```python
from build123d import *

# Parameters (mm, degrees)
F0_R     = 30
F1_DEPTH = 0.5
F2_W     = 30
F2_H     = 1
F4_R     = 30
F4_R_2   = 29.5
F5_DEPTH = 23.5


with BuildPart() as f1:
    # F0 (on Top) → F1 (new body)
    with BuildSketch(Plane.XY):
        Circle(F0_R)
    extrude(amount=-F1_DEPTH)



with BuildPart() as f3:
    # F2 (on Front) → F3 (revolve)
    with BuildSketch(Plane.XZ):
        with Locations((15, -24.5)):
            Rectangle(F2_W, F2_H)
    revolve(axis=Axis((0, 0, -12.5), (0, 0, -1)))


with BuildPart() as f1_1:
    add(f1.part)

    add(f3.part)  # F5 merges F3
    # F4 (on face) → F5 (join, through all)
    with BuildSketch(Plane(origin=(0, 0, -0.5), x_dir=(1, 0, 0), z_dir=(0, 0, -1))):
        Circle(F4_R)
        Circle(F4_R_2, mode=Mode.SUBTRACT)
    extrude(amount=F5_DEPTH)


solid = f1_1.part
```
Build history of the part. All positions in model axes, mm. A direction names the side the tool comes from. Round coordinates to 2 decimals unless told otherwise and drop trailing zeros. Order: outer loops, then holes, each group sorted by start corner. A loop starts at its lowest first (then second) coordinate and runs counter-clockwise, first axis right, second up. Notation, with made-up numbers: (-7, 44) - (30, 44) arc R22 ccw to (30, 63) - close; hole circle Ø8 at (46.25, 45). An arc over 180 degrees is marked (long way). Use a Markdown table: item, result.
1) Saw through at A-A on y = 0. Write the cut outline in (x, z).
Recorded:
| item | result |
|---|---|
| outline | (-30, -25) - (30, -25) - (30, 0) - (-30, 0) - close; hole (-29.5, -24) - (29.5, -24) - (29.5, -0.5) - (-29.5, -0.5) - close |
2) Tool access for faces 1 (the face through (0, 0, -0.5)), 2 (the face through (0, 0, 0)): list every direction of +Z, -Z, +X, -X, +Y, -Y with a clear straight run to the whole face (end or side of a thin tool).
Recorded:
| item | result |
|---|---|
| face 1 | none |
| face 2 | +Z, +X, -X, +Y, -Y |
3) Flat gauge pins, fed straight in: pin 1 Ø6 at (x, z) = (-14.5, -12.5) entering from -Y; pin 2 Ø6 at (y, z) = (10, -19) entering from +X; pin 3 Ø6 at (y, z) = (8, -17.5) entering from -X; pin 4 Ø12 at (x, y) = (-10.5, 8) entering from +Z. Where does each tip first touch, or does it go through?
Recorded:
| item | result |
|---|---|
| pin 1 | stops at y = -27.71 |
| pin 2 | stops at x = 29.17 |
| pin 3 | stops at x = -29.58 |
| pin 4 | stops at z = 0 |
4) Saw through at C-C on z = -5. Write the cut outline in (x, y), and give its area (3 significant figures).
Recorded:
| item | result |
|---|---|
| outline | circle Ø60 at (0, 0); hole circle Ø59 at (0, 0) |
| area | 93.5 mm² |
5) Pull direction Y, two halves, no side cores. Call faces 3 (the face through (0, 0, -25)), 4 (the face through (0, 0, -24)), 5 (the face through (28.14, -8.86, -12.09)): pulls with the +Y half, pulls with the -Y half, needs draft (parallel to the pull), parting line crosses it, or undercut.
Recorded:
| item | result |
|---|---|
| face 3 | needs draft |
| face 4 | undercut |
| face 5 | undercut |
6) Wall check: L1, parallel to X at y = 0, z = -9.5; L2, parallel to Z at x = 19.5, y = -2. Give the ranges that are in metal, low to high.
Recorded:
| item | result |
|---|---|
| L1 | x = -30 to -29.5, 29.5 to 30 |
| L2 | z = -25 to -24, -0.5 to 0 |
